Build history of the part. All positions in model axes, mm. A direction names the side the tool comes from. Coordinates: 2 decimals unless noted, no trailing zeros. Loops run counter-clockwise (first coordinate to the right, second up) from the corner with the lowest first, then second, coordinate; pieces in that order, holes last. Notation, with made-up numbers: (19, 76) - (38, 76) arc R27 ccw to (38, 106) - close; hole circle Ø2 at (22.25, -9). An arc over 180 degrees is marked (long way). One line per item, written item: value.
Autodesk Inventor part; units mm, degrees
ref_plane "YZ Plane" through (0, 0, 0) normal (1, 0, 0) x (0, 1, 0)
ref_plane "XZ Plane" through (0, 0, 0) normal (0, 1, 0) x (-1, 0, 0)
ref_plane "XY Plane" through (0, 0, 0) normal (0, 0, 1) x (1, 0, 0)
sketch "Esquisse1" plane through (0, 0, 0) normal (1, 0, 0) x (0, 1, 0)
  line L0 (0, 22.5) -> (0, -22.5) construction
  line L1 (-7, 22.5) -> (-7, -22.5)
  line L2 (7, -22.5) -> (7, 22.5)
  arc A0 (7, 22.5) -> (-7, 22.5) centre (0, 22.5) ccw
  arc A1 (-7, -22.5) -> (7, -22.5) centre (0, -22.5) ccw
  circle A2 centre (0, 22.5) radius 1.6
  circle A3 centre (0, -22.5) radius 1.6
  point P0 (0, 0)
  dimension "d0" = 45
  dimension "d1" = 3.2
  dimension "d2" = 14
extrude "Extrusion1" add sketch "Esquisse1" along normal blind 4
sketch "Esquisse2" plane through (0, 7, 22.5) normal (0, 1, 0) x (1, 0, 0)
  line L0 (0, 51.1) -> (0, 0)
  line L1 (-18, 24.1) -> (0, 24.1)
  line L2 (0, 24.1) -> (0, 27)
  line L3 (0, 27) -> (-18, 27)
  line L4 (-18, 27) -> (-18, 24.1)
  line L5 (-18, 24.1) -> (0, 27) construction
  line L6 (0, 24.1) -> (-18, 27) construction
  line L7 (-18, 18) -> (0, 18)
  line L8 (0, 18) -> (0, 20.9)
  line L9 (0, 20.9) -> (-18, 20.9)
  line L10 (-18, 20.9) -> (-18, 18)
  line L11 (-18, 18) -> (0, 20.9) construction
  line L12 (0, 18) -> (-18, 20.9) construction
  line L13 (0, 18) -> (0, 27) construction
  line L14 (0, 45) -> (0, 0) construction
  point P0 (0, 22.5)
  point P1 (-9, 25.55)
  point P2 (-9, 19.45)
  point P3 (0, 25.55)
  point P4 (0, 22.5)
  point P5 (0, 24.1)
  point P6 (0, 18)
  point P7 (0, 20.9)
  dimension "d6" = 2.9
  dimension "d7" = 18
  dimension "d10" = 3.2
extrude "Extrusion2" add sketch "Esquisse2" against normal up to surface (14 mm away)
sketch "Esquisse3" plane through (-18, 7, 4.5) normal (0, 0, 1) x (1, 0, 0)
  arc A0 (7, 0) -> (7, -14) centre (7, -7) ccw
  line L0 (0, 0) -> (18, 0) construction
  line L1 (7, 0) -> (18, 0)
  line L2 (18, -14) -> (7, -14)
  line L3 (18, 0) -> (18, 5)
  line L4 (18, 5) -> (-5, 5)
  line L5 (-5, 5) -> (-5, -19)
  line L6 (-5, -19) -> (18, -19)
  line L7 (18, -19) -> (18, -14)
  line L8 (18, 0) -> (18, -14)
  line L9 (0, 0) -> (0, -14) construction
  line L10 (0, -7) -> (-5, -7) construction
  circle A1 centre (7, -7) radius 2.6
  point P0 (18, -7)
  dimension "d11" = 14
  dimension "d12" = 5
  dimension "d16" = 5.2
extrude "Extrusion3" cut sketch "Esquisse3" against normal through all contours A0 L2 L7 L6 L5 L4 L3 L1 | A1
properties part number "support_realsense"
Item 1: Drop flat-ended pins along their axis: P1, Ø6, axis at x = -11, y = 0, coming from the -Z side; P2, Ø4.5, axis at x = -11, y = 0, coming from the +Z side; P3, Ø4, axis at x = -10.5, y = -1, coming from the +Z side; P4, Ø7, axis at y = -2.5, z = 14.5, coming from the -X side. Give the stop position or say it passes through.
Check result:
P1: stops at z = -4.5
P2: passes through
P3: stops at z = 4.5
P4: stops at x = 0
Item 2: Tool access for faces 1 (the face through (-7, 0, -1.6)), 2 (the face through (-18, 0, -3)), 3 (the face through (0, 0, 17)), 4 (the face through (0, 0, -17)): list every direction of +Z, -Z, +X, -X, +Y, -Y with a clear straight run to the whole face (end or side of a thin tool).
Check result:
face 1: -X, +Y, -Y
face 2: +Z, -Z, -X
face 3: +Z, -X, +Y, -Y
face 4: -Z, -X, +Y, -Y
Item 3: Cut at D-D, the plane x = -11.75. Write the cut outline in (y, z).
Check result:
outline: (-6.96, -4.5) - (-2.49, -4.5) - (-2.49, -1.6) - (-6.96, -1.6) - close; (-6.96, 1.6) - (-2.49, 1.6) - (-2.49, 4.5) - (-6.96, 4.5) - close; (2.49, -4.5) - (6.96, -4.5) - (6.96, -1.6) - (2.49, -1.6) - close; (2.49, 1.6) - (6.96, 1.6) - (6.96, 4.5) - (2.49, 4.5) - close
Item 4: Cut at A-A, the plane y = 0. Write the cut outline in (x, z), then the cut area to 3 significant figures.
Check result:
outline: (-18, -4.5) - (-13.6, -4.5) - (-13.6, -1.6) - (-18, -1.6) - close; (-18, 1.6) - (-13.6, 1.6) - (-13.6, 4.5) - (-18, 4.5) - close; (-8.4, -4.5) - (0, -4.5) - (0, -20.9) - (4, -20.9) - (4, 20.9) - (0, 20.9) - (0, 4.5) - (-8.4, 4.5) - (-8.4, 1.6) - (0, 1.6) - (0, -1.6) - (-8.4, -1.6) - close; (0, -29.5) - (4, -29.5) - (4, -24.1) - (0, -24.1) - close; (0, 24.1) - (4, 24.1) - (4, 29.5) - (0, 29.5) - close
area: 285 mm^2
Item 5: Cut at C-C, the plane z = 3. Write the cut outline in (x, y), then the cut area to 3 significant figures.
Check result:
outline: (-11, -7) - (4, -7) - (4, 7) - (-11, 7) arc R7 ccw to start; hole circle Ø5.2 at (-11, 0)
area: 266 mm^2
Item 6: Pull direction Y, two halves, no side cores. Call faces 5 (the face through (1, -7, 0)), 6 (the face through (-7, 0, 1.6)), 7 (the face through (1.972, -0.208, -24.086)), 8 (the face through (1.97, -0.15, 29.5)): released by +Y, released by -Y, zero draft, split by the parting line, or undercut.
Check result:
face 5: released by -Y
face 6: zero draft
face 7: undercut
face 8: split by the parting line
Item 7: Cut at B-B, the plane x = -15. Write the cut outline in (y, z), then the cut area to 3 significant figures.
Check result:
outline: (-5.74, -4.5) - (5.74, -4.5) - (5.74, -1.6) - (-5.74, -1.6) - close; (-5.74, 1.6) - (5.74, 1.6) - (5.74, 4.5) - (-5.74, 4.5) - close
area: 66.6 mm^2
Item 8: Probe probe 1 along Z at (x, y) = (2.35, 0); probe 2 along Z at (x, y) = (-7.75, -1); probe 3 along Y at (x, z) = (-11, 2.25). List the from-to ranges inside material, lowest first. Write a range as from..to.
Check result:
probe 1: z = -29.5..-24.1, -20.9..20.9, 24.1..29.5
probe 2: z = -4.5..-1.6, 1.6..4.5
probe 3: y = -7..-2.6, 2.6..7
